```python
from build123d import *

# Parameters (mm, degrees)
SKETCH003_W       = 37
SKETCH003_H       = 68
PAD002_DEPTH      = 2.6
SKETCH005_R       = 1.5
SKETCH005_R_2     = 4
SKETCH005_W       = 19
SKETCH005_H       = 28.5
POCKET001_DEPTH   = 2.601
SKETCH014_W       = 37
SKETCH014_H       = 68
PAD009_DEPTH      = 2.6
PAD009_DEPTH_BACK = 40.9
SKETCH019_W       = 13
SKETCH019_H       = 8
POCKET005_DEPTH   = 3.501
CHAMFER001_SIZE   = 1.5
SKETCH020_R       = 0.8
SKETCH020_W       = 19
SKETCH020_H       = 12.5
POCKET006_DEPTH   = 3.501
SKETCH034_W       = 14
SKETCH034_H       = 6.5
SKETCH034_H_2     = 2
PAD019_DEPTH      = 6.5
FILLET_R          = 2
CHAMFER_SIZE      = 0.3
CHAMFER002_SIZE   = 2
SKETCH050_W       = 19
SKETCH050_H       = 5
POCKET013_DEPTH   = 2.2


with BuildPart() as part:
    # Sketch003 → Pad002 (new body)
    with BuildSketch(Plane.XY):
        with Locations((18, 33.5)):
            Rectangle(SKETCH003_W, SKETCH003_H)
    extrude(amount=PAD002_DEPTH)

    # Sketch005 → Pocket001 (cut, through all)
    with BuildSketch(Plane.XY):
        with Locations((30.9, 38.4)):
            Circle(SKETCH005_R)
        with Locations((5.1, 38.4)):
            Circle(SKETCH005_R)
        with Locations((5.1, 9.1)):
            Circle(SKETCH005_R)
        with Locations((30.9, 9.1)):
            Circle(SKETCH005_R)
        with Locations((18, 54.25)):
            Circle(SKETCH005_R_2)
        with Locations((18, 26.25)):
            Rectangle(SKETCH005_W, SKETCH005_H)
    extrude(amount=POCKET001_DEPTH, mode=Mode.SUBTRACT)

    # Sketch014 → Pad009 (join, two sides)
    with BuildSketch(Plane.XY) as pad009_sk:
        with BuildLine():
            Line((-0.5, 70.5), (36.5, 70.5))
            ThreePointArc((39.5, 67.5), (38.62132, 69.62132), (36.5, 70.5))
            Line((39.5, 67.5), (39.5, -0.5))
            ThreePointArc((36.5, -3.5), (38.62132, -2.62132), (39.5, -0.5))
            Line((36.5, -3.5), (-0.5, -3.5))
            ThreePointArc((-3.5, -0.5), (-2.62132, -2.62132), (-0.5, -3.5))
            Line((-3.5, -0.5), (-3.5, 67.5))
            ThreePointArc((-0.5, 70.5), (-2.62132, 69.62132), (-3.5, 67.5))
        make_face()
        with Locations((18, 33.5)):
            Rectangle(SKETCH014_W, SKETCH014_H, mode=Mode.SUBTRACT)
    extrude(amount=PAD009_DEPTH)
    extrude(pad009_sk.sketch, amount=-PAD009_DEPTH_BACK)

    # Sketch019 → Pocket005 (cut, through all)
    with BuildSketch(Plane.XZ):
        with Locations((18, -26.225)):
            Rectangle(SKETCH019_W, SKETCH019_H)
    extrude(amount=POCKET005_DEPTH, mode=Mode.SUBTRACT)

    # Chamfer001
    chamfer001_edges = [part.edges().sort_by_distance(p)[0] for p in [
        (3.6, 9.1, 2.6),
        (3.6, 38.4, 2.6),
        (29.4, 38.4, 2.6),
        (29.4, 9.1, 2.6),
    ]]
    chamfer(chamfer001_edges, length=CHAMFER001_SIZE)

    # Sketch020 (on DatumPlane) → Pocket006 (cut, through all)
    with BuildSketch(Plane.XZ.offset(-67)):
        with Locations((11.2, -26.65)):
            Circle(SKETCH020_R)
        with Locations((24.8, -26.65)):
            Circle(SKETCH020_R)
        with Locations((18, -34.65)):
            Rectangle(SKETCH020_W, SKETCH020_H)
    extrude(amount=-POCKET006_DEPTH, mode=Mode.SUBTRACT)

    # Sketch034 → Pad019 (join)
    with BuildSketch(Plane.XY):
        with Locations((18, 64.25)):
            Rectangle(SKETCH034_W, SKETCH034_H)
        with Locations((18, 46)):
            Rectangle(SKETCH034_W, SKETCH034_H_2)
    extrude(amount=-PAD019_DEPTH)

    # Fillet
    fillet_edges = [part.edges().sort_by_distance(p)[0] for p in [
        (39.5, 33.5, 2.6),
    ]]
    fillet(fillet_edges, radius=FILLET_R)

    # Chamfer
    chamfer_edges = [part.edges().sort_by_distance(p)[0] for p in [
        (18, 12, 2.6),
        (8.5, 26.25, 2.6),
        (18, 40.5, 2.6),
        (27.5, 26.25, 2.6),
    ]]
    chamfer(chamfer_edges, length=CHAMFER_SIZE)

    # Chamfer002
    chamfer002_edges = [part.edges().sort_by_distance(p)[0] for p in [
        (14, 54.25, 0),
    ]]
    chamfer(chamfer002_edges, length=CHAMFER002_SIZE)

    # Sketch050 → Pocket013 (cut)
    with BuildSketch(Plane.XY):
        with Locations((18, 9.5)):
            Rectangle(SKETCH050_W, SKETCH050_H)
    extrude(amount=POCKET013_DEPTH, mode=Mode.SUBTRACT)


with BuildPart() as part_1:
    # Body001 placement: moved
    add(part.part.moved(Location((0, 0, 39.4))))


solid = part_1.part
```
Model file for the job. Use its own axes, mm. A direction names the side the tool comes from. Coordinates: 2 decimals unless noted, no trailing zeros. Order: outer loops, then holes, each group sorted by start corner. A loop starts at its lowest first (then second) coordinate and runs counter-clockwise, first axis right, second up. Notation, with made-up numbers: (-18, 25) -> (17, 25) arc R14 ccw to (17, 37) -> close; hole circle Ø10 at (51.25, 1). An arc over 180 degrees is marked (long way). Answer as a JSON object with one key per item and string values. Group by question number.
1) Cut at C-C, the plane x = 5.1. Write the cut outline in (y, z), then the cut area to 3 significant figures.
2) Drill centre lines: L1, parallel to Y at x = 30.9, z = 39.85; L2, parallel to X at y = 9, z = 40; L3, parallel to Y at x = 29.5, z = 19. Where is each one in solid material? Low to high.
3) Pull direction Y, two halves, no side cores. Call faces 5 (the face through (39.5, 34, 20)), 6 (the face through (17.74, -2.9, 41.43)), 7 (the face through (11, 64, 36)): +Y half, -Y half, draft (parallel to the pull), parting line (faces both ways), or undercut.
4) Cut at B-B, the plane y = 9.1. Write the cut outline in (x, z).
5) Cut at D-D, the plane y = 54.25. Write the cut outline in (x, z), then the cut area to 3 significant figures.
6) Cut at A-A, the plane z = 36. Write the cut outline in (x, y).
7) Flat gauge pins, fed straight in: pin 1 (1.8 mm diameter, centred on x = 5.1, y = 38.4, fed in from -Z) (3 decimals); pin 2 (1.6 mm diameter, centred on x = 16.5, y = 45.5, fed in from -Z); pin 3 (1 mm diameter, centred on x = 24.8, z = 12.75, fed in from +Y); pin 4 (2.5 mm diameter, centred on y = 69, z = 5, fed in from +X). Where does each tip first touch, or does it go through?
8) Which spindle directions (+Z, -Z, +X, -X, +Y, -Y) get a long thin tool onto all of the face, cutting with end or side? Do faces 1 (the face through (11.5, -2, 13)), 2 (the face through (18, 10, 41.6)), 3 (the face through (27.5, 69, 5)), 4 (the face through (17.133, 50.345, 41.696)). Say none if no direction does.
Check values:
{
 "1": {"outline": "(-3.5, -1.5) -> (-0.5, -1.5) -> (-0.5, 39.4) -> (7.6, 39.4) -> (7.6, 40.5) -> (6.1, 42) -> (-1.5, 42) arc R2 ccw to (-3.5, 40) -> close; (10.6, 39.4) -> (36.9, 39.4) -> (36.9, 40.5) -> (35.4, 42) -> (12.1, 42) -> (10.6, 40.5) -> close; (39.9, 39.4) -> (67.5, 39.4) -> (67.5, -1.5) -> (70.5, -1.5) -> (70.5, 40) arc R2 ccw to (68.5, 42) -> (41.4, 42) -> (39.9, 40.5) -> close", "area": "416 mm²"},
 "2": {"L1": "y = -3.5 to 7.6, 10.6 to 36.9, 39.9 to 70.5", "L2": "x = -3.5 to 3.6, 6.6 to 8.5, 27.5 to 29.4, 32.4 to 39.5", "L3": "y = -3.5 to -0.5, 67.5 to 70.5"},
 "3": {"face 5": "draft", "face 6": "-Y half", "face 7": "undercut"},
 "4": {"outline": "(-3.5, -1.5) -> (-0.5, -1.5) -> (-0.5, 39.4) -> (3.6, 39.4) -> (3.6, 40.5) -> (2.1, 42) -> (-1.5, 42) arc R2 ccw to (-3.5, 40) -> close; (6.6, 39.4) -> (8.5, 39.4) -> (8.5, 41.6) -> (27.5, 41.6) -> (27.5, 39.4) -> (29.4, 39.4) -> (29.4, 40.5) -> (27.9, 42) -> (8.1, 42) -> (6.6, 40.5) -> close; (32.4, 39.4) -> (36.5, 39.4) -> (36.5, -1.5) -> (39.5, -1.5) -> (39.5, 40) arc R2 ccw to (37.5, 42) -> (33.9, 42) -> (32.4, 40.5) -> close"},
 "5": {"outline": "(-3.5, -1.5) -> (-0.5, -1.5) -> (-0.5, 39.4) -> (12, 39.4) -> (14, 41.4) -> (14, 42) -> (-1.5, 42) arc R2 ccw to (-3.5, 40) -> close; (22, 41.4) -> (24, 39.4) -> (36.5, 39.4) -> (36.5, -1.5) -> (39.5, -1.5) -> (39.5, 40) arc R2 ccw to (37.5, 42) -> (22, 42) -> close", "area": "331 mm²"},
 "6": {"outline": "(-3.5, -0.5) arc R3 ccw to (-0.5, -3.5) -> (36.5, -3.5) arc R3 ccw to (39.5, -0.5) -> (39.5, 67.5) arc R3 ccw to (36.5, 70.5) -> (-0.5, 70.5) arc R3 ccw to (-3.5, 67.5) -> close; (11, 45) -> (25, 45) -> (25, 47) -> (11, 47) -> close; hole (-0.5, -0.5) -> (36.5, -0.5) -> (36.5, 67.5) -> (25, 67.5) -> (25, 61) -> (11, 61) -> (11, 67.5) -> (-0.5, 67.5) -> close"},
 "7": {"pin 1": "passes through", "pin 2": "stops at z = 32.9", "pin 3": "stops at y = -0.5", "pin 4": "stops at x = 39.49"},
 "8": {"face 1": "-Y", "face 2": "-Z", "face 3": "-Z, +Y", "face 4": "+Z, -Z"}
}
